```python
from build123d import *

# Parameters (mm, degrees)
F1_DEPTH = 44.45
F2_R     = 3.175
F3_W     = 19.05
F3_H     = 50.8
F4_DEPTH = 155.1632549


# Not quite as in the source:
# - an extrude ends at something that could not be found from the text; its depth is read off the source's solid


with BuildPart() as f1:
    # F0 (on Front) → F1 (new body)
    with BuildSketch(Plane.XZ):
        with BuildLine():
            Line((9.525, 69.85), (-9.525, 69.85))
            ThreePointArc((-9.525, 69.85), (-20.7503201513, 65.2003201513), (-25.4, 53.975))
            Line((-25.4, 53.975), (-25.4, -53.975))
            ThreePointArc((-25.4, -53.975), (-20.7503201513, -65.2003201513), (-9.525, -69.85))
            Line((-9.525, -69.85), (9.525, -69.85))
            ThreePointArc((9.525, -69.85), (20.7503201513, -65.2003201513), (25.4, -53.975))
            Line((25.4, -53.975), (25.4, 53.975))
            ThreePointArc((25.4, 53.975), (20.7503201513, 65.2003201513), (9.525, 69.85))
        make_face()
    extrude(amount=F1_DEPTH)

    # F2
    f2_edges = [f1.edges().sort_by_distance(p)[0] for p in [
        (0, -44.45, 69.85),
        (20.75032, 0, 65.20032),
        (0, 0, 69.85),
        (-20.75032, 0, 65.20032),
        (-20.75032, -44.45, 65.20032),
        (-25.4, 0, 0),
        (-25.4, -44.45, 0),
        (-20.75032, 0, -65.20032),
        (-20.75032, -44.45, -65.20032),
        (0, 0, -69.85),
        (0, -44.45, -69.85),
        (20.75032, 0, -65.20032),
        (20.75032, -44.45, -65.20032),
        (25.4, 0, 0),
        (25.4, -44.45, 0),
        (20.75032, -44.45, 65.20032),
    ]]
    fillet(f2_edges, radius=F2_R)

    # F3 (on face) → F4 (join, through all)
    with BuildSketch(Plane.YZ.offset(25.4)):
        with Locations((-21.9233557582, 0)):
            Rectangle(F3_W, F3_H)
    extrude(amount=F4_DEPTH)


solid = f1.part
```
Geometry check sheet. Reference: the model listing, model coordinates, mm. A direction names the side the tool comes from. Coordinates: 2 decimals unless noted, no trailing zeros. Write each loop counter-clockwise with the first axis right and the second up, starting at its lowest first coordinate (ties: lowest second). Pieces come first, ordered by that corner, then holes. Notation, with made-up numbers: M 33,61 L 39,61 A11 ccw 39,79 Z; hole C -10.75,-24 d7. An arc over 180 degrees is marked long. Use one line per item in the form item = value. Start each with the question number.
1) Section check B-B on z = 19. Enter the section's corners in (x, y) (3 decimals), and give its area (3 significant figures).
2) Section check C-C on x = 148.5. Enter the section's corners in (y, z), and give its area (3 significant figures).
3) Section check A-A on y = -15. Enter the section's corners in (x, z) (3 decimals), and give its area (3 significant figures).
4) Go/stop test with flat-tipped pins: pin 1 Ø15 at (x, y) = (84, -19) entering from -Z; pin 2 Ø5.5 at (x, y) = (85, -17.5) entering from +Z; pin 3 Ø2 at (x, z) = (38, 10.5) entering from -Y. Record where each tip stops, or that it passes through.
5) Set-up check for faces 1 (the flat face through (102, -31.448, 0)), 2 (the flat face through (102, -22, -25.4)), 3 (the flat face through (102, -12.398, 0)): record each of +Z, -Z, +X, -X, +Y, -Y from which the full face is reachable in a straight line by a thin tool's end or side.
6) Section check D-D on y = -36.5. Enter the section's corners in (x, z) (3 decimals), and give its area (3 significant figures).
7) Thickness scan on probe 1 along X at (y, z) = (-38, 9); probe 2 along Y at (x, z) = (62, 10.5). Record the ranges inside material, lowest first. Write a range as from..to.
Responses:
q1.outline = M -25.4,-41.275 A3.175 ccw -22.225,-44.45 L 22.225,-44.45 A3.175 ccw 25.4,-41.275 L 25.4,-31.448 L 180.563,-31.448 L 180.563,-12.398 L 25.4,-12.398 L 25.4,-3.175 A3.175 ccw 22.225,0 L -22.225,0 A3.175 ccw -25.4,-3.175 Z
q1.area = 5,210 mm2
q2.outline = M -31.45,-25.4 L -12.4,-25.4 L -12.4,25.4 L -31.45,25.4 Z
q2.area = 968 mm2
q3.outline = M -25.4,-53.975 A15.875 ccw -9.525,-69.85 L 9.525,-69.85 A15.875 ccw 25.4,-53.975 L 25.4,-25.4 L 180.563,-25.4 L 180.563,25.4 L 25.4,25.4 L 25.4,53.975 A15.875 ccw 9.525,69.85 L -9.525,69.85 A15.875 ccw -25.4,53.975 Z
q3.area = 14,800 mm2
q4.pin_1 = -25.4
q4.pin_2 = 25.4
q4.pin_3 = -31.45
q5.face_1 = +Z, -Z, +X, -Y
q5.face_2 = -Z, +X, +Y, -Y
q5.face_3 = +Z, -Z, +X, +Y
q6.outline = M -25.4,-53.975 A15.875 ccw -9.525,-69.85 L 9.525,-69.85 A15.875 ccw 25.4,-53.975 L 25.4,53.975 A15.875 ccw 9.525,69.85 L -9.525,69.85 A15.875 ccw -25.4,53.975 Z
q6.area = 6,880 mm2
q7.probe_1 = -25.4..25.4
q7.probe_2 = -31.45..-12.4
